Autodesk Fusion 360 part; units mm, degrees
sketch "Sketch1" plane through (0, 0, 0) normal (0, 1, 0) x (1, 0, 0)
  line L0 (20, -19) -> (-20, -19)
  line L1 (-20, -19) -> (-20, 19)
  line L2 (-20, 19) -> (20, 19)
  line L3 (20, 19) -> (20, -19)
  line L4 (20, -19) -> (-20, 19) construction
  line L5 (-20, -19) -> (20, 19) construction
  line L6 (125, -19) -> (-125, -19)
  line L7 (-125, -19) -> (-125, 19)
  line L8 (-125, 19) -> (125, 19)
  line L9 (125, 19) -> (125, -19)
  line L10 (125, -19) -> (-125, 19) construction
  line L11 (-125, -19) -> (125, 19) construction
  dimension "d1" = 40
  dimension "d2" = 38
  dimension "d25" = 250
  dimension "d26" = 38
extrude "Extrude1" add sketch "Sketch1" along normal blind 30 contours L0 L1 L2 L3 L6 L8
sketch "Sketch3" plane through (0, 0, -19) normal (0, 0, -1) x (-1, 0, 0)
  line L0 (-20, 0) -> (20, 0)
  line L1 (20, 0) -> (20, 30)
  line L2 (-20, 30) -> (-20, 0)
  circle A0 centre (0, 20) radius 10
  circle A1 centre (0, 20) radius 2.7
  line L3 (20, 30) -> (-20, 30)
  dimension "d13" = 5.4
extrude "Extrude3" cut sketch "Sketch3" against normal blind 60 contours A1
extrude "Extrude4" cut sketch "Sketch3" against normal blind 6 contours A0
extrude "Extrude5" cut sketch "Sketch3" against normal blind 6 from surface at -32 contours A0
extrude "Extrude6" add sketch "Sketch1" along normal blind 10 from surface at 30
chamfer "Chamfer2" distance 5 angle 45 4 edges at (0, 40, 19) (0, 40, -19) (0, 0, 19) (0, 0, -19)
chamfer "Chamfer3" distance 12 angle 45 2 edges at (20, 0, 0) (-20, 0, 0)
extrude "Extrude7" cut sketch "Sketch1" along normal blind 5 contours L0 L1 L2 L3 L6 L8
sketch "Sketch5" plane through (0, 40, 0) normal (0, -1, 0) x (1, 0, 0)
  line L0 (-9.9736, 7.5643) -> (-9.9736, -7.9957)
  line L1 (-9.9736, -7.9957) -> (10.2882, -7.9957)
  line L2 (10.2882, -7.9957) -> (10.2882, 7.5643)
  line L3 (10.2882, 7.5643) -> (-9.9736, 7.5643)
  circle A0 centre (-8.5238, 6.1446) radius 0.9796
  circle A1 centre (1.4942, 6.1953) radius 0.9537
  circle A2 centre (8.9673, 6.2107) radius 1.0098
  circle A3 centre (-1.0564, 6.2266) radius 0.9892
  circle A4 centre (7.6339, -5.3368) radius 1.5084
  circle A5 centre (-6.0639, 6.1567) radius 0.9903
  circle A6 centre (3.9566, 6.1712) radius 0.9784
  circle A7 centre (6.4638, 6.2006) radius 0.9737
  circle A8 centre (-3.4927, 6.169) radius 0.9564
  circle A9 centre (-7.4269, -5.3596) radius 1.4324
  line L4 (10.5, 8.5) -> (-10.5, 8.5)
  line L5 (-10.5, 8.5) -> (-10.5, -8.5)
  line L6 (-10.5, -8.5) -> (10.5, -8.5)
  line L7 (10.5, -8.5) -> (10.5, 8.5)
  line L8 (10.5, 8.5) -> (-10.5, -8.5) construction
  line L9 (-10.5, 8.5) -> (10.5, -8.5) construction
  line L10 (125, -14) -> (-125, -14)
  line L11 (-125, -14) -> (-125, 14)
  line L12 (-125, 14) -> (125, 14)
  line L13 (125, 14) -> (125, -14)
  dimension "d33" = 21
  dimension "d34" = 17
extrude "Extrude8" cut sketch "Sketch5" along normal blind 5 contours A4 | A9
extrude "Extrude9" cut sketch "Sketch5" along normal blind 0.5 contours L0 L1 L2 L3 | A0 | A1 | A2 | A3 | A5 | A6 | A7 | A8 | L4 L5 L6 L7
Input: part model. Units: mm. Frame: model coordinates. A direction names the side the tool comes from. Round coordinates to 2 decimals unless told otherwise and drop trailing zeros. Loops run counter-clockwise (first coordinate to the right, second up) from the corner with the lowest first, then second, coordinate; pieces in that order, holes last.
1) Set-up query: faces 4 (the flat face through (72, 30, 0)), 5 (the flat face through (-2.1, 17.9, 13)), 6 (the flat face through (-73, 30, 0)). Return all of +Z, -Z, +X, -X, +Y, -Y with unobstructed straight access to the full face (end or side cutting, diameter ignored); none if empty.
Ans:
face 4: +Z, -Z, +X, -Y
face 5: +Z
face 6: +Z, -Z, -X, -Y
2) Pin query (flat end, axial travel): pin 1 (20 mm diameter, centred on y = 16.5, z = 9, fed in from +X); pin 2 (1.5 mm diameter, centred on x = 7.5, z = -5, fed in from +Y); pin 3 (8 mm diameter, centred on x = -96, y = 24, fed in from +Z); pin 4 (8.5 mm diameter, centred on x = 0, y = 20, fed in from +Z). Return the tip coordinate at first contact, or that it passes through.
Ans:
pin 1: stops at x = 20
pin 2: stops at y = 35
pin 3: passes through
pin 4: stops at z = 13
3) Material intervals for line 1 (X direction, y = 20, z = -17); line 2 (X direction, y = 37.5, z = -6.5); line 3 (Y direction, x = 28.5, z = 0), sorted ascending.
Ans:
line 1: x = -20 to -10, 10 to 20
line 2: x = -125 to -8.29, -6.56 to 6.67, 8.59 to 125
line 3: y = 30 to 40
4) Section query A-A on x = 0. Return the cut outline in (y, z), plus the area to 3 significant figures.
Ans:
outline: (5, -19) - (10, -19) - (10, -13) - (17.3, -13) - (17.3, 13) - (10, 13) - (10, 19) - (5, 19) - close; (22.7, -13) - (30, -13) - (30, -19) - (35, -19) - (40, -14) - (40, -8.5) - (39.5, -8.5) - (39.5, 8.5) - (40, 8.5) - (40, 14) - (35, 19) - (30, 19) - (30, 13) - (22.7, 13) - close
area: 916 mm2
5) Section query C-C on z = 6. Return the cut outline in (x, y).
Ans:
outline: (-125, 30) - (-20, 30) - (-20, 12) - (-13, 5) - (13, 5) - (20, 12) - (20, 30) - (125, 30) - (125, 40) - (10.5, 40) - (10.5, 39.5) - (-10.5, 39.5) - (-10.5, 40) - (-125, 40) - close; hole circle Ø5.4 at (0, 20)
6) Section query B-B on y = 20. Return the cut outline in (x, z).
Ans:
outline: (-20, -19) - (-10, -19) - (-10, -13) - (-2.7, -13) - (-2.7, 13) - (-10, 13) - (-10, 19) - (-20, 19) - close; (2.7, -13) - (10, -13) - (10, -19) - (20, -19) - (20, 19) - (10, 19) - (10, 13) - (2.7, 13) - close
7) Section query D-D on x = -45. Return the cut outline in (y, z), plus the area to 3 significant figures.
Ans:
outline: (30, -19) - (35, -19) - (40, -14) - (40, 14) - (35, 19) - (30, 19) - close
area: 355 mm2
8) Pull-direction query (Y, two-part tool) for faces 1 (the flat face through (-2, 38, 16)), 2 (the flat face through (-16, 8, 0)), 3 (the cylindrical face through (1.302, 29.915, 15.958)); classes: released by +Y, released by -Y, zero draft, split by the parting line, or undercut.
Ans:
face 1: released by +Y
face 2: released by -Y
face 3: undercut
